from build123d import *

# Parameters (mm, degrees)
ESQUISSE1_W             = 60
ESQUISSE1_H             = 36
BOSS_EXTRU_1_DEPTH      = 12
ENL_V_MAT_EXTRU_1_REACH = 38.986
ESQUISSE2_R             = 11.5
TROU_TARAUD_M51_D       = 4.2
CHANFREIN1_SIZE         = 1


with BuildPart() as part:
    # Esquisse1 → Boss.-Extru.1 (new body)
    with BuildSketch(Plane.XY):
        Rectangle(ESQUISSE1_W, ESQUISSE1_H)
    extrude(amount=BOSS_EXTRU_1_DEPTH)

    # Esquisse2 → Enlèv. mat.-Extru.1 (cut, up to next)
    with BuildSketch(Plane.XY.offset(12), mode=Mode.PRIVATE) as enl_v_mat_extru_1_sk1:
        Circle(ESQUISSE2_R)
    enl_v_mat_extru_1_tool1 = extrude(enl_v_mat_extru_1_sk1.sketch, amount=-ENL_V_MAT_EXTRU_1_REACH, mode=Mode.PRIVATE) & part.part
    add(enl_v_mat_extru_1_tool1.solids().sort_by_distance((0, 0, 12))[0], mode=Mode.SUBTRACT)

    # Trou taraudé M51 (through all)
    with Locations(Plane.XY.offset(12)):
        with Locations((-25, 0), (25, 0)):
            Hole(TROU_TARAUD_M51_D / 2)

    # Chanfrein1
    chanfrein1_edges = [part.edges().sort_by_distance(p)[0] for p in [
        (30, 0, 12),
        (0, 18, 12),
        (-11.5, 0, 12),
        (-11.5, 0, 0),
        (-30, 0, 12),
        (0, 18, 0),
        (30, 0, 0),
        (0, -18, 0),
        (-30, 0, 0),
        (0, -18, 12),
        (-30, 18, 6),
        (30, 18, 6),
        (30, -18, 6),
        (-30, -18, 6),
    ]]
    chamfer(chanfrein1_edges, length=CHANFREIN1_SIZE)


solid = part.part
Input: part model. Units: mm. Frame: model coordinates. Give positions to 0.01 mm unless a question says otherwise; leave off trailing zeros. Write each loop counter-clockwise with the first axis right and the second up, starting at its lowest first coordinate (ties: lowest second). Pieces come first, ordered by that corner, then holes.
Q1. Section D-D, the plane x = -24. Output: boundary loops of the cut face in (y, z).
Q2. Section C-C, the plane x = 25. Output: boundary loops of the cut face in (y, z), plus the area to 3 significant figures.
Q3. Pull-direction query (X, two-part tool) for faces 1 (the face through (-1.5, 11.4, 6.1)), 2 (the face through (30, 0, 6)), 3 (the face through (-27.003, 0.631, 5.916)), 4 (the face through (-30, 0, 6)); classes: pulls with the +X half, pulls with the -X half, needs draft (parallel to the pull), parting line crosses it, or undercut.
Q4. Section A-A, the plane y = 0. Output: boundary loops of the cut face in (x, z).
Q5. Material intervals for probe 1 along Y at (x, z) = (25, 7); probe 2 along Y at (x, z) = (0, 5.75); probe 3 along X at (y, z) = (-9.5, 5.75), sorted ascending.
Q6. Section B-B, the plane z = 4.25. Output: boundary loops of the cut face in (x, y), plus the area to 3 significant figures.
Filled in:
1. outline: (-18, 1) - (-17, 0) - (-1.85, 0) - (-1.85, 12) - (-17, 12) - (-18, 11) - close; (1.85, 0) - (17, 0) - (18, 1) - (18, 11) - (17, 12) - (1.85, 12) - close
2. outline: (-18, 1) - (-17, 0) - (-2.1, 0) - (-2.1, 12) - (-17, 12) - (-18, 11) - close; (2.1, 0) - (17, 0) - (18, 1) - (18, 11) - (17, 12) - (2.1, 12) - close
2. area: 380 mm2
3. face 1: undercut
3. face 2: pulls with the +X half
3. face 3: undercut
3. face 4: pulls with the -X half
4. outline: (-30, 1) - (-29, 0) - (-27.1, 0) - (-27.1, 12) - (-29, 12) - (-30, 11) - close; (-22.9, 0) - (-12.5, 0) - (-11.5, 1) - (-11.5, 11) - (-12.5, 12) - (-22.9, 12) - close; (11.5, 1) - (12.5, 0) - (22.9, 0) - (22.9, 12) - (12.5, 12) - (11.5, 11) - close; (27.1, 0) - (29, 0) - (30, 1) - (30, 11) - (29, 12) - (27.1, 12) - close
5. probe 1: y = -18 to -2.1, 2.1 to 18
5. probe 2: y = -18 to -11.5, 11.5 to 18
5. probe 3: x = -30 to -6.48, 6.48 to 30
6. outline: (-30, -17) - (-29, -18) - (29, -18) - (30, -17) - (30, 17) - (29, 18) - (-29, 18) - (-30, 17) - close; hole circle Ø4.2 at (-25, 0); hole circle Ø23 at (0, 0); hole circle Ø4.2 at (25, 0)
6. area: 1,710 mm2
